from build123d import *

# Parameters (mm, degrees)
SKETCH_1_W          = 42.2
SKETCH_1_H          = 42.2
EXTRUDE_1_DEPTH     = 10
SKETCH_2_R          = 1.6
SKETCH_2_R_2        = 3
CUT_EXTRUDE_1_DEPTH = 6
SKETCH_3_R          = 11
CUT_EXTRUDE_2_DEPTH = 2
SKETCH_4_R          = 5
CUT_EXTRUDE_3_DEPTH = 11
SKETCH_5_R          = 1.3
CUT_EXTRUDE_4_DEPTH = 11


with BuildPart() as part:
    # 草图1 → 凸台-拉伸1 (new body)
    with BuildSketch(Plane.XY):
        Rectangle(SKETCH_1_W, SKETCH_1_H)
    extrude(amount=EXTRUDE_1_DEPTH)

    # 草图2 → 切除-拉伸1 (cut)
    with BuildSketch(Plane(origin=(0, 0, 0), x_dir=(-1, 0, 0), z_dir=(0, 0, -1))):
        with Locations((12.5, 0)):
            Circle(SKETCH_2_R)
        with Locations((0, -12.5)):
            Circle(SKETCH_2_R)
        with Locations((-12.5, 0)):
            Circle(SKETCH_2_R)
        with Locations((0, 12.5)):
            Circle(SKETCH_2_R)
        with Locations((-15.5, 15.5)):
            Circle(SKETCH_2_R_2)
        with Locations((15.5, 15.5)):
            Circle(SKETCH_2_R_2)
        with Locations((15.5, -15.5)):
            Circle(SKETCH_2_R_2)
        with Locations((-15.5, -15.5)):
            Circle(SKETCH_2_R_2)
    extrude(amount=-CUT_EXTRUDE_1_DEPTH, mode=Mode.SUBTRACT)

    # 草图3 → 切除-拉伸2 (cut)
    with BuildSketch(Plane.XY.offset(10)):
        Circle(SKETCH_3_R)
    extrude(amount=-CUT_EXTRUDE_2_DEPTH, mode=Mode.SUBTRACT)

    # 草图4 → 切除-拉伸3 (cut, through all)
    with BuildSketch(Plane(origin=(0, 0, 0), x_dir=(-1, 0, 0), z_dir=(0, 0, -1))):
        Circle(SKETCH_4_R)
    extrude(amount=-CUT_EXTRUDE_3_DEPTH, mode=Mode.SUBTRACT)

    # 草图5 → 切除-拉伸4 (cut, through all)
    with BuildSketch(Plane.XY.offset(10)):
        with Locations((15.5, -15.5)):
            Circle(SKETCH_5_R)
        with Locations((-15.5, -15.5)):
            Circle(SKETCH_5_R)
        with Locations((-15.5, 15.5)):
            Circle(SKETCH_5_R)
        with Locations((15.5, 15.5)):
            Circle(SKETCH_5_R)
    extrude(amount=-CUT_EXTRUDE_4_DEPTH, mode=Mode.SUBTRACT)


solid = part.part
Verification items for the finished model (mm, model axes). A direction names the side the tool comes from. Give positions to 0.01 mm unless a question says otherwise; leave off trailing zeros. Write each loop counter-clockwise with the first axis right and the second up, starting at its lowest first coordinate (ties: lowest second). Pieces come first, ordered by that corner, then holes.
(1) Material ranges on line 1 (Y direction, x = 15.5, z = 8.7); line 2 (Y direction, x = 15.5, z = 1.2); line 3 (Y direction, x = 0, z = 9.55), recorded low to high.
(2) Cross-section at D-D (z = 2.75). State how many separate pieces and enclosed holes the cut face has, plus the area to 3 significant figures.
(3) Cross-section at A-A (x = 15.5). Enter the section's corners in (y, z), plus the area to 3 significant figures.
(4) Access from +Z, -Z, +X, -X, +Y, -Y to the whole of each face (thin tool, end or side, straight path). Record for faces 1 (the face through (-5, 5, 0)), 2 (the face through (2, -5, 8)), 3 (the face through (-12, 0, 6)).
(5) Mould release check, pull along Y, two halves, no side actions. Record for faces 4 (the face through (-16.458, 16.379, 8.028)), 5 (the face through (0, 21.1, 5)), 6 (the face through (-10, -9, 10)): +Y half, -Y half, draft (parallel to the pull), parting line (faces both ways), or undercut.
(6) Cross-section at B-B (z = 9). Enter the section's corners in (x, y).
(7) Cross-section at C-C (x = 0). Enter the section's corners in (y, z).
(8) Gauge pin test, flat ends, axial feed: pin 1 (3.5 mm diameter, centred on x = 15.5, y = -15.5, fed in from +Z); pin 2 (11 mm diameter, centred on x = 0.5, y = -1, fed in from +Z); pin 3 (5.5 mm diameter, centred on x = 15.5, y = 15.5, fed in from -Z). Record the tip position at first contact, or that the pin passes through.
Worked out:
1. line 1: y = -21.1 to -16.8, -14.2 to 14.2, 16.8 to 21.1
1. line 2: y = -21.1 to -18.5, -12.5 to 12.5, 18.5 to 21.1
1. line 3: y = -21.1 to -11, 11 to 21.1
2. separate pieces: 1
2. enclosed holes: 9
2. area: 1,560 mm2
3. outline: (-21.1, 0) - (-18.5, 0) - (-18.5, 6) - (-16.8, 6) - (-16.8, 10) - (-21.1, 10) - close; (-14.2, 6) - (-12.5, 6) - (-12.5, 0) - (12.5, 0) - (12.5, 6) - (14.2, 6) - (14.2, 10) - (-14.2, 10) - close; (16.8, 6) - (18.5, 6) - (18.5, 0) - (21.1, 0) - (21.1, 10) - (16.8, 10) - close
3. area: 329 mm2
4. face 1: -Z, +X, -X, +Y, -Y
4. face 2: +Z
4. face 3: -Z
5. face 4: undercut
5. face 5: +Y half
5. face 6: draft
6. outline: (-21.1, -21.1) - (21.1, -21.1) - (21.1, 21.1) - (-21.1, 21.1) - close; hole circle Ø2.6 at (-15.5, -15.5); hole circle Ø2.6 at (-15.5, 15.5); hole circle Ø22 at (0, 0); hole circle Ø2.6 at (15.5, -15.5); hole circle Ø2.6 at (15.5, 15.5)
7. outline: (-21.1, 0) - (-14.1, 0) - (-14.1, 6) - (-10.9, 6) - (-10.9, 0) - (-5, 0) - (-5, 8) - (-11, 8) - (-11, 10) - (-21.1, 10) - close; (5, 0) - (10.9, 0) - (10.9, 6) - (14.1, 6) - (14.1, 0) - (21.1, 0) - (21.1, 10) - (11, 10) - (11, 8) - (5, 8) - close
8. pin 1: stops at z = 10
8. pin 2: stops at z = 8
8. pin 3: stops at z = 6
